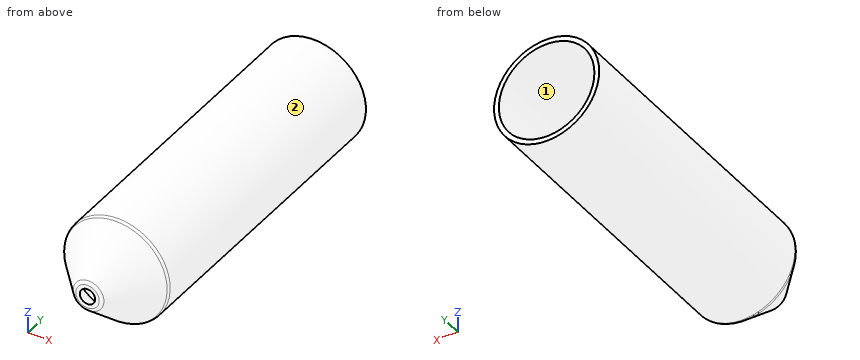
```python
from build123d import *

# Parameters (mm, degrees)
FILLET1_R = 2
FILLET3_R = 2


with BuildPart() as part:
    # Sketch1 → Revolve1 (revolve)
    with BuildSketch(Plane.XY):
        Polygon((-22, 0), (-22, -130.727940469), (-5.828821955, -150), (-3.218007376, -150), (-20, -130), (-20, 0), align=None)
    revolve(axis=Axis((0, 0, 0), (0, -1, 0)))

    # Fillet1
    fillet1_edges = [part.edges().sort_by_distance(p)[0] for p in [
        (22, -130.727940469, 0),
    ]]
    fillet(fillet1_edges, radius=FILLET1_R)

    # Fillet3
    fillet3_edges = [part.edges().sort_by_distance(p)[0] for p in [
        (5.828821955, -150, 0),
    ]]
    fillet(fillet3_edges, radius=FILLET3_R)


solid = part.part
```
The listing builds one solid part. Answer for the finished solid, in the listing's coordinates (mm). Face numbers are marked on the shaded views. Give positions to 0.01 mm unless a question says otherwise; leave off trailing zeros. Order: outer loops, then holes, each group sorted by start corner. A loop starts at its lowest first (then second) coordinate and runs counter-clockwise, first axis right, second up. Notation, with made-up numbers: (12.5, 20.5) - (35.5, 20.5) arc R12 ccw to (35.5, 39.5) - close; hole circle Ø5 at (49, -4). An arc over 180 degrees is marked (long way). Answer in a Markdown table with one row per item. Add a question column.
Q1. The part is cut by section A-A (y = -58.5). Determine the outline of the cut face in (x, z), then the cut area to 3 significant figures.
Q2. For a pull along X with two mould halves and no side action, classify the marked faces 1 and 2 as released by +X, released by -X, zero draft, split by the parting line, or undercut.
Q3. Find the intervals of material crossed by line 1 along X through (y, z) = (-56, 0); line 2 along Z through (x, y) = (5.5, -133), in increasing order. Write a range as [from, to].
Q4. Given P1, Ø5, axis at x = 11, y = -117, coming from the +Z side; P2, Ø2, axis at y = -102.5, z = -6.5, coming from the +X side; P3, Ø12, axis at x = 11.5, z = 2.5, coming from the -Y side, each flat-ended and moving along its own axis, determine where each tip first touches the part or whether it passes through.
Determined:
| question | item | result |
|---|---|---|
| 1 | outline | circle Ø44 at (0, 0); hole circle Ø40 at (0, 0) |
| 1 | area | 264 mm² |
| 2 | face 1 | undercut |
| 2 | face 2 | split by the parting line |
| 3 | line 1 | x = [-22, -20], [20, 22] |
| 3 | line 2 | z = [-19.33, -16.6], [16.6, 19.33] |
| 4 | P1 | stops at z = 20.29 |
| 4 | P2 | stops at x = 21.3 |
| 4 | P3 | stops at y = -149.8 |
